Autodesk Inventor part; units mm, degrees
ref_plane "YZ Plane" through (0, 0, 0) normal (1, 0, 0) x (0, 1, 0)
ref_plane "XZ Plane" through (0, 0, 0) normal (0, 1, 0) x (-1, 0, 0)
ref_plane "XY Plane" through (0, 0, 0) normal (0, 0, 1) x (1, 0, 0)
sketch "Sketch1" plane through (0, 0, 0) normal (1, 0, 0) x (0, 1, 0)
  line L0 (0, 0) -> (0, 25.4)
  line L1 (0, 0) -> (13.97, 0)
  arc A0 (13.97, 0) -> (0, 25.4) centre (-21.4675, -2.9489) ccw
  line L2 (0, 0) -> (0, 15.748)
  line L3 (0, 15.748) -> (8.7805, 15.748)
  dimension "d0" = 25.4
  dimension "d1" = 13.97
  dimension "d2" = 35.56
  dimension "d3" = 15.748
revolve "Revolution1" add sketch "Sketch1" angle 360 about axis through (0, 0, 0) along (0, 1, 0)
sketch "Sketch4" plane through (0, 0, 0) normal (0, -1, 0) x (1, 0, 0)
  line L0 (0, 0) -> (12.897, 0)
  line L1 (12.897, 0) -> (12.897, 21.8821)
  circle A0 centre (0, 0) radius 25.4
  line L2 (12.897, 21.8821) -> (38.6124, 21.8821)
  line L3 (38.6124, 21.8821) -> (38.6124, -32.9808)
  line L4 (38.6124, -32.9808) -> (12.897, -32.9808)
  line L5 (12.897, -32.9808) -> (12.897, 21.8821)
  dimension "d12" = 21.8821
extrude "Extrusion3" cut sketch "Sketch4" against normal through all contours L1 A0 L5 | L2 L3 L4 L5 A0 picked at (14.3084, 13.5451)
sketch "Sketch5" plane through (12.897, 0, 21.8821) normal (1, 0, 0) x (0, 0, -1)
  line L0 (21.8821, 0) -> (21.8821, 5.08)
  circle A0 centre (21.8821, 5.08) radius 1.27
  dimension "d15" = 5.08
  dimension "d16" = 2.54
extrude "Extrusion4" cut sketch "Sketch5" against normal blind 2.54
sketch "Sketch6" plane through (0, 0, 0) normal (0, -1, 0) x (1, 0, 0)
  circle A0 centre (0, 0) radius 1.27
  dimension "d19" = 2.54
extrude "Extrusion5" cut sketch "Sketch6" against normal blind 2.54
properties part number "camera side"
Here's how the part is built. I have some questions about the finished solid (model axes, mm). A direction names the side the tool comes from. Coordinates: 2 decimals unless noted, no trailing zeros. Answer as CSV lines item,"result".
Item 1: For pin 1 (1 mm diameter, centred on x = 5.5, y = 9, fed in from +Z); pin 2 (4 mm diameter, centred on x = -3, y = 9, fed in from +Z); pin 3 (1.5 mm diameter, centred on x = -10, z = 17, fed in from +Y), each with a flat end and sliding along its axis, tell me the tip position at first contact or that it passes through.
Results found:
pin 1,"z = 15.25"
pin 2,"z = 18.13"
pin 3,"y = 6.53"
Item 2: On a 3-axis mill with a long thin cutter (end or side, diameter ignored), from which of +Z, -Z, +X, -X, +Y, -Y can I reach the whole of each face in a straight line? I mean faces 1 (the face through (-6, 0, 0)), 2 (the face through (10.357, 5, 0)), 3 (the face through (-0.17, 1.25, 1.26)). Say none if no direction works.
Results found:
face 1,"+Z, -Z, +X, -X, -Y"
face 2,"+X"
face 3,"-Y"
Item 3: We'd pull the mould along Z, two halves only. Please class faces 4 (the face through (11.64, 3.84, 0.28)), 5 (the face through (0, 2.54, 0)), 6 (the face through (12.897, 3, 0)): +Z half, -Z half, draft (parallel to the pull), parting line (faces both ways), or undercut.
Results found:
face 4,"undercut"
face 5,"undercut"
face 6,"draft"
Item 4: If I drill on line 1 (Z direction, x = 0, y = 1.4); line 2 (Z direction, x = 0, y = 2); line 3 (Y direction, x = 11, z = 0), over which ranges is the centre line in solid material (lowest first)?
Results found:
line 1,"-24.28 to -1.27, 1.27 to 24.28"
line 2,"-23.77 to -1.27, 1.27 to 23.77"
line 3,"0 to 3.81, 6.35 to 11.24"
